Source: CAD feature listing. Evaluate the final solid. Frame: model axes, mm. Face numbers are marked on the shaded views. A direction names the side the tool comes from. Give positions to 0.01 mm unless a question says otherwise; leave off trailing zeros. Loops run counter-clockwise (first coordinate to the right, second up) from the corner with the lowest first, then second, coordinate; pieces in that order, holes last.
```python
from build123d import *

# Parameters (mm, degrees)
F1_DEPTH    = 20
F3_DEPTH    = 5.1
F4_R        = 5
F5_R        = 1
F6_R        = 1
F7_T1_DEPTH = 20
F7_T4_ANGLE = 70
F7_T6_ANGLE = 70


# Not quite as in the source:
# - a fillet or chamfer that OpenCascade refuses, or shapes differently, is made with other operations: its cross-section is extruded or revolved along the edge and cut away or added


with BuildPart() as f1:
    # F0 (on Top) → F1 (new body)
    with BuildSketch(Plane.XY):
        with BuildLine():
            Line((30, 0), (0, 0))
            ThreePointArc((0, 0), (-9, -9), (0, -18))
            ThreePointArc((0, -18), (2, -16), (0, -14))
            ThreePointArc((0, -14), (-5, -9), (0, -4))
            Line((0, -4), (26.0285742974, -4))
            Line((26.0285742974, -4), (33.7580712171, -25.2366182506))
            ThreePointArc((33.7580712171, -25.2366182506), (37.0264387656, -26.7606830681), (38.5505035831, -23.4923155196))
            Line((38.5505035831, -23.4923155196), (30, 0))
        make_face()
    extrude(amount=F1_DEPTH)

    # F2 (on face) → F3 (cut, through all)
    with BuildSketch(Plane(origin=(26.4906666468, 9.6418141453, 0), x_dir=(-0.3420201433, 0.9396926208, 0), z_dir=(0.9396926208, 0.3420201433, 0))):
        with BuildLine():
            ThreePointArc((-19.9606042998, 15), (-20.2534975186, 15.7071067812), (-20.9606042998, 16))
            Line((-20.9606042998, 16), (-22.9606042998, 16))
            ThreePointArc((-22.9606042998, 16), (-23.667711081, 15.7071067812), (-23.9606042998, 15))
            Line((-23.9606042998, 15), (-23.9606042998, 5))
            ThreePointArc((-23.9606042998, 5), (-23.667711081, 4.2928932188), (-22.9606042998, 4))
            Line((-22.9606042998, 4), (-20.9606042998, 4))
            ThreePointArc((-20.9606042998, 4), (-20.2534975186, 4.2928932188), (-19.9606042998, 5))
            Line((-19.9606042998, 5), (-19.9606042998, 15))
        make_face()
        with BuildLine():
            ThreePointArc((-28.0606042998, 15), (-28.3534975186, 15.7071067812), (-29.0606042998, 16))
            Line((-29.0606042998, 16), (-31.0606042998, 16))
            ThreePointArc((-31.0606042998, 16), (-31.767711081, 15.7071067812), (-32.0606042998, 15))
            Line((-32.0606042998, 15), (-32.0606042998, 5))
            ThreePointArc((-32.0606042998, 5), (-31.767711081, 4.2928932188), (-31.0606042998, 4))
            Line((-31.0606042998, 4), (-29.0606042998, 4))
            ThreePointArc((-29.0606042998, 4), (-28.3534975186, 4.2928932188), (-28.0606042998, 5))
            Line((-28.0606042998, 5), (-28.0606042998, 15))
        make_face()
    extrude(amount=-F3_DEPTH, mode=Mode.SUBTRACT)

    # F4
    f4_edges = [f1.edges().sort_by_distance(p)[0] for p in [
        (26.028574, -4, 10),
    ]]
    fillet(f4_edges, radius=F4_R)

    # F5
    f5_edges = [f1.edges().sort_by_distance(p)[0] for p in [
        (15, 0, 20),
        (11.263768, -4, 20),
        (25.395419, -4.90424, 20),
        (-5, -9, 20),
        (30.492035, -16.263259, 20),
        (2, -16, 20),
        (37.026439, -26.760683, 20),
        (-9, -9, 20),
        (34.275252, -11.746158, 20),
    ]]
    fillet(f5_edges, radius=F5_R)

    # F6
    f6_edges = [f1.edges().sort_by_distance(p)[0] for p in [
        (11.263768, -4, 0),
        (25.395419, -4.90424, 0),
        (-5, -9, 0),
        (30.492035, -16.263259, 0),
        (2, -16, 0),
        (37.026439, -26.760683, 0),
        (-9, -9, 0),
        (34.275252, -11.746158, 0),
        (15, 0, 0),
    ]]
    fillet(f6_edges, radius=F6_R)

    # F7: fillet of radius 5 on 1 edges, made by hand

    # F7_s2 → F7_t1 (cut)
    with BuildSketch(Plane.XY):
        with BuildLine():
            ThreePointArc((31.1982351897, -3.290954605), (29.3668444907, -0.9042397786), (26.497693671, 0.0004))
            Line((26.497693671, 0.0004), (26.497693671, 0.5006211803))
            ThreePointArc((26.497693671, 0.5006211803), (28.2488468355, 0.5002211803), (30, 0.5002211803))
            Line((30, 0.5002211803), (30.4700541519, 0.1710857198))
            ThreePointArc((30.4700541519, 0.1710857198), (31.0689838082, -1.4744599868), (31.6682893415, -3.1198688852))
            Line((31.6682893415, -3.1198688852), (31.1982351897, -3.290954605))
        make_face()
    extrude(amount=F7_T1_DEPTH, mode=Mode.SUBTRACT)

    # F7_s3 → F7_t4 (revolve, cut)
    with BuildSketch(Plane.YZ.offset(26.497693671)):
        with BuildLine():
            ThreePointArc((-0.9996, 0), (-0.2924932188, 0.2928932188), (0.0004, 1))
            Line((0.0004, 1), (0.0004, 0))
            Line((0.0004, 0), (-0.9996, 0))
        make_face()
    revolve(axis=Axis((26.497693671, -5.0018118027, 0), (0, 0, -1)), revolution_arc=F7_T4_ANGLE, mode=Mode.SUBTRACT)

    # F7_s5 → F7_t6 (revolve, cut)
    with BuildSketch(Plane(origin=(4.7071926658, -12.9329055584, 0), x_dir=(0, 0, 1), z_dir=(0.3420201433, -0.9396926208, 0))):
        with BuildLine():
            ThreePointArc((20, -27.1911786236), (19.7071067812, -27.8982854048), (19, -28.1911786236))
            Line((19, -28.1911786236), (20, -28.1911786236))
            Line((20, -28.1911786236), (20, -27.1911786236))
        make_face()
    revolve(axis=Axis((26.497693671, -5.0018118027, 20), (0, 0, 1)), revolution_arc=F7_T6_ANGLE, mode=Mode.SUBTRACT)


solid = f1.part
```
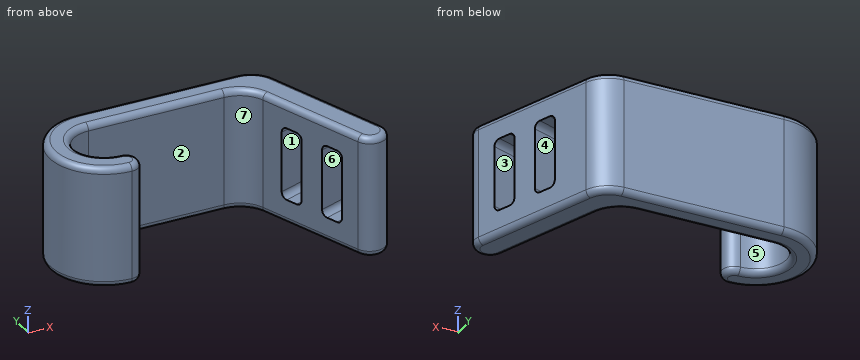
(1) Section A-A, the plane z = 11.25. Return the cut outline in (x, y).
A:
outline: (0, -18) arc R2 ccw to (0, -14) arc R5 cw to (0, -4) - (22.53, -4) arc R5 cw to (27.23, -7.29) - (28.53, -10.86) - (33.32, -9.12) - (31.18, -3.23) arc R5 ccw to (26.56, 0) - (0, 0) arc R9 ccw to start; (29.89, -14.62) - (31.3, -18.47) - (36.09, -16.73) - (34.69, -12.87) - close; (32.66, -22.23) - (33.76, -25.24) arc R2.55 ccw to (38.55, -23.49) - (37.46, -20.49) - close
(2) First-contact query: pin 1 (5.5 mm diameter, centred on x = 15, z = 10.5, fed in from -Y); pin 2 (3 mm diameter, centred on x = 30.5, y = -4, fed in from +Z); pin 3 (2 mm diameter, centred on y = -22, z = 18, fed in from +X); pin 4 (6 mm diameter, centred on y = -18.5, z = 5, fed in from +X). Flat tips, straight axial feed; report the tip coordinate or a pass-through.
A:
pin 1: stops at y = -4
pin 2: stops at z = 20
pin 3: stops at x = 38.37
pin 4: stops at x = 37.83
(3) Reachability of the marked faces 4, 5, 6 and 7 from +Z, -Z, +X, -X, +Y, -Y: full face, straight path, thin tool, end or side. Return the list, or none.
A:
face 4: none
face 5: +Z, -Z
face 6: +X
face 7: +Z, -Z, -Y
(4) Ray query, line 1 along Y through (x, z) = (20, 13.25); line 2 along X through (y, z) = (-8.5, 8); line 3 along Y through (x, z) = (-0.5, 6). Return the intervals inside material, ascending.
A:
line 1: y = -4 to 0
line 2: x = -8.99 to -4.97, 27.67 to 33.09
line 3: y = -17.99 to -13.97, -4.03 to -0.01
(5) Section C-C, the plane z = 2.75. Return the cut outline in (x, y).
A:
outline: (0, -18) arc R2 ccw to (0, -14) arc R5 cw to (0, -4) - (22.53, -4) arc R5 cw to (27.23, -7.29) - (33.76, -25.24) arc R2.55 ccw to (38.55, -23.49) - (31.18, -3.23) arc R5 ccw to (26.56, 0) - (0, 0) arc R9 ccw to start
(6) Section B-B, the plane x = 18.5. Return the cut outline in (y, z), then the cut area to 3 significant figures.
A:
outline: (-4, 1) arc R1 ccw to (-3, 0) - (-1, 0) arc R1 ccw to (0, 1) - (0, 19) arc R1 ccw to (-1, 20) - (-3, 20) arc R1 ccw to (-4, 19) - close
area: 79.1 mm2
(7) Mould query, pull axis X, two halves, no side actions, for the marked faces 1, 2 and 3. Classes: pulls with the +X half, pulls with the -X half, needs draft (parallel to the pull), parting line crosses it, or undercut.
A:
face 1: pulls with the +X half
face 2: undercut
face 3: pulls with the -X half
